The listing builds one solid part. Answer for the finished solid, in the listing's coordinates (mm). A direction names the side the tool comes from. Round coordinates to 2 decimals unless told otherwise and drop trailing zeros. Write each loop counter-clockwise with the first axis right and the second up, starting at its lowest first coordinate (ties: lowest second). Pieces come first, ordered by that corner, then holes. Notation, with made-up numbers: M 69.25,19 L 121.25,19 A30 cw 121.25,47 Z; hole C -4.75,47 d2. An arc over 180 degrees is marked long. One line per item, written item: value. Start each with the question number.
(1) For a pull along X with two mould halves and no side action, classify faces 1 (the flat face through (64, -28, 0)), 2 (the cylindrical face through (178.734, -29.938, 0.986)) as released by +X, released by -X, zero draft, split by the parting line, or undercut.
(2) Section D-D (z = 1.35) is taken. State how many separate pieces and enclosed holes the cut face has, plus the area to 3 significant figures.
(3) Section A-A (x = 131) is taken. Determine the outline of the cut face in (y, z), plus the area to 3 significant figures.
(4) Section C-C (x = 34) is taken. Determine the outline of the cut face in (y, z), plus the area to 3 significant figures.
(5) Section B-B (y = -58) is taken. Determine the outline of the cut face in (x, z).
(6) Consider probe 1 along X at (y, z) = (-16.5, 1); probe 2 along X at (y, z) = (-50.5, 0.1); probe 3 along Y at (x, z) = (28, 0.4). Determine where each line is inside the solid, lowest interval first.
(7) For faces 3 (the cylindrical face through (66.109, -39.078, 0.986)), 4 (the cylindrical face through (-10.543, -29.274, 0.986)), determine the directions among +Z, -Z, +X, -X, +Y, -Y from which every point of the face is accessible in a straight line to the end or side of a thin tool.
```python
from build123d import *

# Parameters (mm, degrees)
SKETCH_1_W                    = 230
SKETCH_1_H                    = 100
EXTRUDE_1_DEPTH               = 2
SKETCH_3_W                    = 2.2
SKETCH_3_H                    = 50
SKETCH_3_W_2                  = 30
SKETCH_3_H_2                  = 5
CUT_EXTRUDE_2_DEPTH           = 2
CUT_EXTRUDE_2_DEPTH_BACK      = 2
CUT_EXTRUDE_3_DEPTH           = 2
CUT_EXTRUDE_3_DEPTH_BACK      = 2
SKETCH_5_R                    = 2.25
CUT_EXTRUDE_8_DEPTH           = 2
CUT_EXTRUDE_8_TAPER           = 1
CUT_EXTRUDE_8_OTHER_WAY_DEPTH = 2


with BuildPart() as part:
    # Sketch 1 → Extrude 1 (new body)
    with BuildSketch(Plane.XY):
        with Locations((65.955242642, -29.076013845)):
            Rectangle(SKETCH_1_W, SKETCH_1_H)
    extrude(amount=EXTRUDE_1_DEPTH)

    # Sketch 3 → Cut-Extrude 2 (cut, two sides)
    with BuildSketch(Plane.XY) as cut_extrude_2_sk:
        with Locations((-32.644757358, -29.076013845)):
            Rectangle(SKETCH_3_W, SKETCH_3_H)
        with Locations((13.455242642, -14.076013845)):
            Rectangle(SKETCH_3_W_2, SKETCH_3_H_2)
        with BuildLine():
            Line((-1.544757358, -20.076013845), (28.455242642, -20.076013845))
            ThreePointArc((28.455242642, -20.076013845), (37.455242642, -29.076013845), (28.455242642, -38.076013845))
            Line((28.455242642, -38.076013845), (-1.544757358, -38.076013845))
            ThreePointArc((-1.544757358, -38.076013845), (-10.544757358, -29.076013845), (-1.544757358, -20.076013845))
        make_face()
        with Locations((13.455242642, -44.076013845)):
            Rectangle(SKETCH_3_W_2, SKETCH_3_H_2)
        with Locations((118.455242642, -44.076013845)):
            Rectangle(SKETCH_3_W_2, SKETCH_3_H_2)
        with BuildLine():
            Line((133.455242642, -38.076013845), (103.455242642, -38.076013845))
            ThreePointArc((103.455242642, -38.076013845), (94.455242642, -29.076013845), (103.455242642, -20.076013845))
            Line((103.455242642, -20.076013845), (133.455242642, -20.076013845))
            ThreePointArc((133.455242642, -20.076013845), (142.455242642, -29.076013845), (133.455242642, -38.076013845))
        make_face()
        with Locations((118.455242642, -14.076013845)):
            Rectangle(SKETCH_3_W_2, SKETCH_3_H_2)
        with Locations((164.555242642, -29.076013845)):
            Rectangle(SKETCH_3_W, SKETCH_3_H)
    extrude(amount=CUT_EXTRUDE_2_DEPTH, mode=Mode.SUBTRACT)
    extrude(cut_extrude_2_sk.sketch, amount=-CUT_EXTRUDE_2_DEPTH_BACK, mode=Mode.SUBTRACT)

    # Sketch 4 → Cut-Extrude 3 (cut, two sides)
    with BuildSketch(Plane.XY) as cut_extrude_3_sk:
        with BuildLine():
            Line((43.955242642, -46.076013845), (43.955242642, -79.076013845))
            Line((43.955242642, -79.076013845), (52.455242642, -79.076013845))
            Line((52.455242642, -79.076013845), (52.455242642, -46.076013845))
            ThreePointArc((52.455242642, -46.076013845), (48.205242642, -41.826013845), (43.955242642, -46.076013845))
        make_face()
        with BuildLine():
            Line((58.955242642, -46.076013845), (58.955242642, -79.076013845))
            Line((58.955242642, -79.076013845), (72.955242642, -79.076013845))
            Line((72.955242642, -79.076013845), (72.955242642, -46.076013845))
            ThreePointArc((72.955242642, -46.076013845), (65.955242642, -39.076013845), (58.955242642, -46.076013845))
        make_face()
        with BuildLine():
            Line((79.455242642, -46.076013845), (79.455242642, -79.076013845))
            Line((79.455242642, -79.076013845), (87.955242642, -79.076013845))
            Line((87.955242642, -79.076013845), (87.955242642, -46.076013845))
            ThreePointArc((87.955242642, -46.076013845), (83.705242642, -41.826013845), (79.455242642, -46.076013845))
        make_face()
    extrude(amount=CUT_EXTRUDE_3_DEPTH, mode=Mode.SUBTRACT)
    extrude(cut_extrude_3_sk.sketch, amount=-CUT_EXTRUDE_3_DEPTH_BACK, mode=Mode.SUBTRACT)

    # Sketch 5 → Cut-Extrude 8 (cut)
    with BuildSketch(Plane.XY):
        with Locations((-44.744757358, -29.076013845)):
            Circle(SKETCH_5_R)
        with Locations((176.655242642, -29.076013845)):
            Circle(SKETCH_5_R)
    extrude(amount=-CUT_EXTRUDE_8_DEPTH, taper=CUT_EXTRUDE_8_TAPER, mode=Mode.SUBTRACT)

    # Sketch 5 → Cut-Extrude 8 other way (cut)
    with BuildSketch(Plane.XY):
        with Locations((-44.744757358, -29.076013845)):
            Circle(SKETCH_5_R)
        with Locations((176.655242642, -29.076013845)):
            Circle(SKETCH_5_R)
    extrude(amount=CUT_EXTRUDE_8_OTHER_WAY_DEPTH, mode=Mode.SUBTRACT)


solid = part.part
```
Recorded:
1. face 1: zero draft
1. face 2: undercut
2. separate pieces: 1
2. enclosed holes: 10
2. area: 19,400 mm2
3. outline: M -79.08,0 L -46.58,0 L -46.58,2 L -79.08,2 Z; M -41.58,0 L -38.08,0 L -38.08,2 L -41.58,2 Z; M -20.08,0 L -16.58,0 L -16.58,2 L -20.08,2 Z; M -11.58,0 L 20.92,0 L 20.92,2 L -11.58,2 Z
3. area: 144 mm2
4. outline: M -79.08,0 L -36.17,0 L -36.17,2 L -79.08,2 Z; M -21.99,0 L 20.92,0 L 20.92,2 L -21.99,2 Z
4. area: 172 mm2
5. outline: M -49.04,0 L 43.96,0 L 43.96,2 L -49.04,2 Z; M 52.46,0 L 58.96,0 L 58.96,2 L 52.46,2 Z; M 72.96,0 L 79.46,0 L 79.46,2 L 72.96,2 Z; M 87.96,0 L 180.96,0 L 180.96,2 L 87.96,2 Z
6. probe 1: x = -49.04 to -33.74, -31.54 to -1.54, 28.46 to 103.46, 133.46 to 163.46, 165.66 to 180.96
6. probe 2: x = -49.04 to -33.74, -31.54 to 43.96, 52.46 to 58.96, 72.96 to 79.46, 87.96 to 163.46, 165.66 to 180.96
6. probe 3: y = -79.08 to -46.58, -41.58 to -38.08, -20.08 to -16.58, -11.58 to 20.92
7. face 3: +Z, -Z, -Y
7. face 4: +Z, -Z
